from build123d import *

# Parameters (mm, degrees)
SKIZZE1_W                       = 20.3
SKIZZE1_H                       = 20.3
AUFSATZ_LINEAR_AUSTRAGEN1_DEPTH = 10
VERRUNDUNG1_R                   = 0.2
VERRUNDUNG2_R                   = 2.5
SKIZZE2_R                       = 2.3
SCHNITT_LINEAR_AUSTRAGEN1_DEPTH = 44.53748385
SKETCH1_R                       = 3.75
CUT_EXTRUDE1_DEPTH              = 1.6
CUT_EXTRUDE2_START              = -36.3
SKETCH1_2_R                     = 3.75
CUT_EXTRUDE2_DEPTH              = 1.6
FASE2_SIZE                      = 0.5


with BuildPart() as part:
    # Skizze1 → Aufsatz-Linear austragen1 (new body)
    with BuildSketch(Plane.XY):
        with BuildLine():
            Line((14.727440375, 18.95), (-14.727440375, 18.95))
            ThreePointArc((-14.727440375, 18.95), (-16.970562748, 16.970562748), (-18.95, 14.727440375))
            Line((-18.95, 14.727440375), (-18.95, -14.727440375))
            ThreePointArc((-18.95, -14.727440375), (-16.970562748, -16.970562748), (-14.727440375, -18.95))
            Line((-14.727440375, -18.95), (14.727440375, -18.95))
            ThreePointArc((14.727440375, -18.95), (16.970562748, -16.970562748), (18.95, -14.727440375))
            Line((18.95, -14.727440375), (18.95, 14.727440375))
            ThreePointArc((18.95, 14.727440375), (16.970562748, 16.970562748), (14.727440375, 18.95))
        make_face()
        Rectangle(SKIZZE1_W, SKIZZE1_H, mode=Mode.SUBTRACT)
    extrude(amount=AUFSATZ_LINEAR_AUSTRAGEN1_DEPTH)

    # Verrundung1
    verrundung1_edges = [part.edges().sort_by_distance(p)[0] for p in [
        (10.15, -10.15, 5),
        (10.15, 10.15, 5),
        (-10.15, 10.15, 5),
        (-10.15, -10.15, 5),
    ]]
    fillet(verrundung1_edges, radius=VERRUNDUNG1_R)

    # Verrundung2
    verrundung2_edges = [part.edges().sort_by_distance(p)[0] for p in [
        (18.95, 14.727440375, 5),
        (18.95, -14.727440375, 5),
        (14.727440375, -18.95, 5),
        (-14.727440375, -18.95, 5),
        (-18.95, -14.727440375, 5),
        (-18.95, 14.727440375, 5),
        (-14.727440375, 18.95, 5),
        (14.727440375, 18.95, 5),
    ]]
    fillet(verrundung2_edges, radius=VERRUNDUNG2_R)

    # Skizze2 → Schnitt-Linear austragen1 (cut, through all)
    with BuildSketch(Plane(origin=(18.95, 0, 0), x_dir=(0, 0, -1), z_dir=(1, 0, 0))):
        with Locations(Location((-5, 0, 0), (0, 0, 90))):
            Circle(SKIZZE2_R)
    extrude(amount=-SCHNITT_LINEAR_AUSTRAGEN1_DEPTH, mode=Mode.SUBTRACT)

    # Sketch1 → Cut-Extrude1 (cut)
    with BuildSketch(Plane.ZY.offset(18.95)):
        with Locations(Location((5, 0, 0), (0, 0, 270))):
            Circle(SKETCH1_R)
    extrude(amount=-CUT_EXTRUDE1_DEPTH, mode=Mode.SUBTRACT)

    # Sketch1<2> → Cut-Extrude2 (cut)
    with BuildSketch(Plane.ZY.offset(18.95).offset(CUT_EXTRUDE2_START)):
        with Locations(Location((5, 0, 0), (0, 0, 270))):
            Circle(SKETCH1_2_R)
    extrude(amount=-CUT_EXTRUDE2_DEPTH, mode=Mode.SUBTRACT)

    # Fase2
    fase2_edges = [part.edges().sort_by_distance(p)[0] for p in [
        (-10.15, -2.3, 5),
        (10.15, -2.3, 5),
        (-17.35, -2.3, 5),
        (17.35, -2.3, 5),
        (0, -10.15, 0),
        (0, -10.15, 10),
        (10.15, 0, 0),
        (10.15, 0, 10),
        (-10.15, 0, 0),
        (-10.15, 0, 10),
        (0, 10.15, 0),
        (0, 10.15, 10),
        (10.091421356, -10.091421356, 0),
        (10.091421356, -10.091421356, 10),
        (-10.091421356, -10.091421356, 0),
        (-10.091421356, -10.091421356, 10),
        (-10.091421356, 10.091421356, 0),
        (-10.091421356, 10.091421356, 10),
        (10.091421356, 10.091421356, 0),
        (10.091421356, 10.091421356, 10),
        (0, 18.95, 0),
        (0, 18.95, 10),
        (16.970562748, 16.970562748, 0),
        (18.95, 0, 0),
        (16.970562748, -16.970562748, 0),
        (0, -18.95, 0),
        (-16.970562748, -16.970562748, 0),
        (-18.95, 0, 0),
        (-16.970562748, 16.970562748, 0),
        (-14.700425655, 18.798614139, 0),
        (-18.798614139, 14.700425655, 0),
        (-18.798614139, -14.700425655, 0),
        (-14.700425655, -18.798614139, 0),
        (14.700425655, -18.798614139, 0),
        (18.798614139, -14.700425655, 0),
        (18.798614139, 14.700425655, 0),
        (14.700425655, 18.798614139, 0),
        (16.970562748, 16.970562748, 10),
        (-16.970562748, 16.970562748, 10),
        (-18.95, 0, 10),
        (-16.970562748, -16.970562748, 10),
        (0, -18.95, 10),
        (16.970562748, -16.970562748, 10),
        (18.95, 0, 10),
        (-14.700425655, 18.798614139, 10),
        (-18.798614139, 14.700425655, 10),
        (-18.798614139, -14.700425655, 10),
        (-14.700425655, -18.798614139, 10),
        (14.700425655, -18.798614139, 10),
        (18.798614139, -14.700425655, 10),
        (18.798614139, 14.700425655, 10),
        (14.700425655, 18.798614139, 10),
    ]]
    chamfer(fase2_edges, length=FASE2_SIZE)


solid = part.part
Check sheet for the modelled part. Datum: model origin and axes. Units: mm. A direction names the side the tool comes from. Give positions to 0.01 mm unless a question says otherwise; leave off trailing zeros. Write each loop counter-clockwise with the first axis right and the second up, starting at its lowest first coordinate (ties: lowest second). Pieces come first, ordered by that corner, then holes. Notation, with made-up numbers: (85, 87) -> (132, 87) arc R28 cw to (132, 126) -> close; hole circle Ø4 at (26.25, 4). An arc over 180 degrees is marked (long way). One line per item, written item: value. Start each with the question number.
Item 1: Section check A-A on y = 9. Record the cut outline in (x, z), then the cut area to 3 significant figures.
Item 2: Tool access check on faces 5 (the flat face through (17.35, 3, 5)), 6 (the cylindrical face through (-13.707, -0.499, 2.755)), 7 (the flat face through (-17.35, 3, 5)). Record the directions out of +Z, -Z, +X, -X, +Y, -Y that give a thin tool (end or side, any length) a straight path to the whole face; none if there is none.
Item 3: Material ranges on probe 1 along X at (y, z) = (9, 9.5); probe 2 along Z at (x, y) = (18, 0), recorded low to high. Write a range as from..to.
Item 4: Section check D-D on y = 0. State how many separate pieces and enclosed holes the cut face has, then the cut area to 3 significant figures.
Item 5: Gauge pin test, flat ends, axial feed: pin 1 (3 mm diameter, centred on y = -0.5, z = 4.5, fed in from -X); pin 2 (1 mm diameter, centred on y = -1.5, z = 7, fed in from -X); pin 3 (4 mm diameter, centred on y = 0, z = 4, fed in from +X); pin 4 (2 mm diameter, centred on y = -1.5, z = 5, fed in from +X). Record the tip position at first contact, or that the pin passes through.
Item 6: Draft check along Y on faces 1 (the flat face through (-10.15, -2.4, 6.9)), 2 (the cylindrical face through (-18.8, -14.7, 5.1)), 3 (the flat face through (10.15, -2.4, 6.9)), 4 (the cylindrical face through (16.99, 16.95, 4.94)). Enter one of: +Y half, -Y half, draft (parallel to the pull), parting line (faces both ways), or undercut.
Results list:
1. outline: (-18.95, 0.5) -> (-18.45, 0) -> (-10.65, 0) -> (-10.15, 0.5) -> (-10.15, 9.5) -> (-10.65, 10) -> (-18.45, 10) -> (-18.95, 9.5) -> close; (10.15, 0.5) -> (10.65, 0) -> (18.45, 0) -> (18.95, 0.5) -> (18.95, 9.5) -> (18.45, 10) -> (10.65, 10) -> (10.15, 9.5) -> close
1. area: 175 mm²
2. face 5: +X
2. face 6: +X, -X
2. face 7: -X
3. probe 1: -18.95..-10.15, 10.15..18.95
3. probe 2: 0..1.25, 8.75..10
4. separate pieces: 4
4. enclosed holes: 0
4. area: 83.8 mm²
5. pin 1: through
5. pin 2: x = -17.35
5. pin 3: x = 17.35
5. pin 4: x = 17.05
6. face 1: undercut
6. face 2: -Y half
6. face 3: undercut
6. face 4: +Y half
